Part model, mm, in its own coordinate system. Face numbers are marked on the shaded views. Give positions to 0.01 mm unless a question says otherwise; leave off trailing zeros. Write each loop counter-clockwise with the first axis right and the second up, starting at its lowest first coordinate (ties: lowest second). Pieces come first, ordered by that corner, then holes. Notation, with made-up numbers: M 42.25,8 L 66.25,8 A31 cw 66.25,37 Z; hole C 22,48 d8. An arc over 180 degrees is marked long. Use CSV: the item, a comma, the result in double quotes. Start each with the question number.
1. Drill centre lines: line 1 along X through (y, z) = (1.65, 0); line 2 along Y through (x, z) = (-12.5, 34.5); line 3 along Y through (x, z) = (-15.5, -12). Where is each one in solid material? Low to high. Write a range as from..to.
2. Band-saw the part on B-B, the plane x = 0. List the corners of the cut face in (y, z).
3. Band-saw the part on A-A, the plane z = 0. List the corners of the cut face in (x, y).
4. Mould opens along Z. For the marked faces 1 and 2 say: pulls with the +Z half, pulls with the -Z half, needs draft (parallel to the pull), parting line crosses it, or undercut.
5. Drop flat-ended pins along their axis: pin 1 Ø4 at (y, z) = (6.5, -30.5) entering from +X; pin 2 Ø5 at (x, y) = (23, 8.5) entering from -Z; pin 3 Ø5 at (y, z) = (6.5, 5) entering from +X; pin 4 Ø14 at (x, z) = (0, -53.8) entering from -Y. Give the stop position or say it passes through.
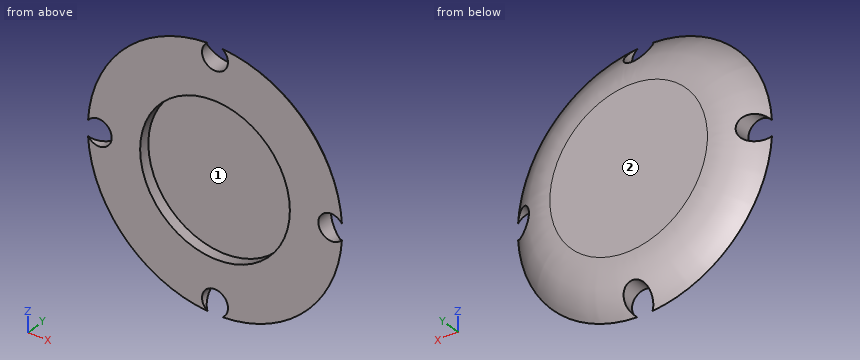
from build123d import *

# Parameters (mm, degrees)
CROQUIS1_R              = 58.8
SALIENTE_EXTRUIR1_DEPTH = 10
REDONDEO1_R             = 30
CROQUIS2_R              = 34.614627086
CORTAR_EXTRUIR1_DEPTH   = 5
CROQUIS3_R              = 6
CORTAR_EXTRUIR2_DEPTH   = 32


with BuildPart() as part:
    # Croquis1 → Saliente-Extruir1 (new body)
    with BuildSketch(Plane(origin=(0, 0, 0), x_dir=(1, 0, 0), z_dir=(0, 1, 0))):
        with Locations(Location((0, 0, 0), (0, 0, 270))):
            Circle(CROQUIS1_R)
    extrude(amount=SALIENTE_EXTRUIR1_DEPTH)

    # Redondeo1
    # the kernel refuses this fillet: 30 mm, written as the material it takes off along each edge
    with BuildSketch(Plane(origin=(0, 10, 0), x_dir=(0, 0, 1), z_dir=(-1, 0, 0))) as redondeo1_piece_1:
        with BuildLine():
            CenterArc((36.439320225, -30), REDONDEO1_R, 41.810314896, 48.189685104)
            Line((36.439320225, 0), (36.439320225, 0.6))
            Line((36.439320225, 0.6), (58.8, 0.6))
            Line((58.8, 0.6), (59.4, 0))
            ThreePointArc((59.4, 0), (59.4, -5), (59.247213595, -9.6))
            Line((59.247213595, -9.6), (58.8, -10))
        make_face()
    revolve(axis=Axis((0, 10, 0), (0, 1, 0)), mode=Mode.SUBTRACT)

    # Croquis2 → Cortar-Extruir1 (cut)
    with BuildSketch(Plane(origin=(0, 0, 0), x_dir=(-1, 0, 0), z_dir=(0, -1, 0))):
        with Locations(Location((0, 0, 0), (0, 0, 90))):
            Circle(CROQUIS2_R)
    extrude(amount=-CORTAR_EXTRUIR1_DEPTH, mode=Mode.SUBTRACT)

    # Croquis3 → Cortar-Extruir2 (cut)
    with BuildSketch(Plane(origin=(0, 0, 0), x_dir=(-1, 0, 0), z_dir=(0, -1, 0))):
        with Locations((0, -53.8)):
            Circle(CROQUIS3_R)
        with Locations((-53.8, 0)):
            Circle(CROQUIS3_R)
        with Locations((0, 53.8)):
            Circle(CROQUIS3_R)
        with Locations((53.8, 0)):
            Circle(CROQUIS3_R)
    extrude(amount=-CORTAR_EXTRUIR2_DEPTH, mode=Mode.SUBTRACT)


solid = part.part
Output:
1,line 1,"x = -47.8..-34.61, 34.61..47.8"
1,line 2,"y = 0..10"
1,line 3,"y = 5..10"
2,outline,"M 0,-47.8 L 7.77,-47.8 A30 ccw 10,-36.44 L 10,36.44 A30 ccw 7.77,47.8 L 0,47.8 L 0,34.61 L 5,34.61 L 5,-34.61 L 0,-34.61 Z"
3,outline,"M -47.8,0 L -34.61,0 L -34.61,5 L 34.61,5 L 34.61,0 L 47.8,0 L 47.8,7.77 A30 ccw 36.44,10 L -36.44,10 A30 ccw -47.8,7.77 Z"
4,face 1,"undercut"
4,face 2,"needs draft"
5,pin 1,"stops at x = 44.52"
5,pin 2,"stops at z = -46.13"
5,pin 3,"stops at x = 53.82"
5,pin 4,"stops at y = 0"
